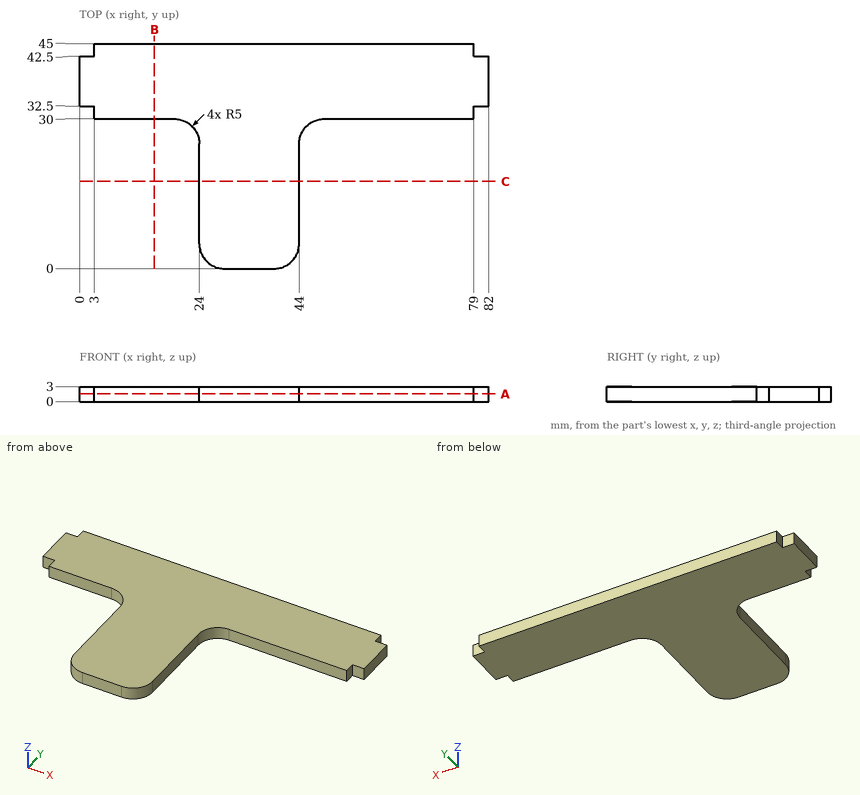
Study the drawing (mm; zero at the part's minimum x, y, z) and answer. Round coordinates to 2 decimals unless told otherwise and drop trailing zeros. Loops run counter-clockwise (first coordinate to the right, second up) from the corner with the lowest first, then second, coordinate; pieces in that order, holes last. Notation, with made-up numbers: M -22.5,-35.75 L -8.5,-35.75 A27 cw -8.5,0.25 Z; hole C -20.75,75.5 d5. An arc over 180 degrees is marked long. One line per question, with ' | ' between items.
Q1. Find section B-B, the plane x = 15. Give the vertices of the cut face in (y, z), then the cut area to 3 significant figures.
Conclusion:
outline: M 30,0 L 45,0 L 45,3 L 30,3 Z | area: 45.0 mm2
Q2. Each of these flat-tipped pins is pushed along its axis until it touches: pin 1 Ø1.5 at (x, z) = (11, 2.5) entering from -Y; pin 2 Ø1.5 at (x, z) = (80.5, 2) entering from +Y; pin 3 Ø1.5 at (x, z) = (19.5, 1) entering from -Y; pin 4 Ø10 at (x, y) = (53, 12.5) entering from +Z. Where does it stop, or does it pass through?
Conclusion:
pin 1: stops at y = 30 | pin 2: stops at y = 42.5 | pin 3: stops at y = 29.84 | pin 4: passes through
Q3. Find section C-C, the plane y = 17.5. Give the vertices of the cut face in (x, z), then the cut area to 3 significant figures.
Conclusion:
outline: M 24,0 L 44,0 L 44,3 L 24,3 Z | area: 60.0 mm2
Q4. Consider line 1 along Y through (x, z) = (7, 0.45); line 2 along X through (y, z) = (21.5, 1.55); line 3 along X through (y, z) = (31, 2.85). Determine where each line is inside the solid, lowest interval first. Write a range as from..to.
Conclusion:
line 1: y = 30..45 | line 2: x = 24..44 | line 3: x = 3..79
Q5. Find section A-A, the plane z = 1.55. Give the vertices of the cut face in (x, y).
Conclusion:
outline: M 0,32.5 L 3,32.5 L 3,30 L 19,30 A5 cw 24,25 L 24,5 A5 ccw 29,0 L 39,0 A5 ccw 44,5 L 44,25 A5 cw 49,30 L 79,30 L 79,32.5 L 82,32.5 L 82,42.5 L 79,42.5 L 79,45 L 3,45 L 3,42.5 L 0,42.5 Z
